```python
from build123d import *

# Parameters (mm, degrees)
SKETCH3_W           = 156.772980402
SKETCH3_H           = 60
BOSS_EXTRUDE6_DEPTH = 12
CUT_EXTRUDE1_REACH  = 14
SKETCH4_R           = 2.25
CUT_EXTRUDE2_REACH  = 14
SKETCH6_R           = 3.25
SKETCH7_R           = 3.5
CUT_EXTRUDE3_DEPTH  = 5
SKETCH8_R           = 5
CUT_EXTRUDE4_DEPTH  = 7
CUT_EXTRUDE5_REACH  = 14
SKETCH9_R           = 2.75


with BuildPart() as part:
    # Sketch3 → Boss-Extrude6 (new body)
    with BuildSketch(Plane(origin=(-27.52701042, 0, 0), x_dir=(0, 0, 1), z_dir=(0, 1, 0))):
        with Locations((-23.695908121, 17.809773729)):
            Rectangle(SKETCH3_W, SKETCH3_H)
    extrude(amount=BOSS_EXTRUDE6_DEPTH)

    # Sketch4 → Cut-Extrude1 (cut, up to next)
    with BuildSketch(Plane(origin=(0, 12, 0), x_dir=(1, 0, 0), z_dir=(0, 1, 0)), mode=Mode.PRIVATE) as cut_extrude1_sk1:
        with Locations((-1.126993796, -19.304091879)):
            Circle(SKETCH4_R)
    cut_extrude1_tool1 = extrude(cut_extrude1_sk1.sketch, amount=-CUT_EXTRUDE1_REACH, mode=Mode.PRIVATE) & part.part
    add(cut_extrude1_tool1.solids().sort_by_distance((-1.126994, 12, 19.304092))[0], mode=Mode.SUBTRACT)
    # Sketch4 → Cut-Extrude1 (cut, up to next)
    with BuildSketch(Plane(origin=(0, 12, 0), x_dir=(1, 0, 0), z_dir=(0, 1, 0)), mode=Mode.PRIVATE) as cut_extrude1_sk2:
        with Locations((-19.127096376, -19.304091879)):
            Circle(SKETCH4_R)
    cut_extrude1_tool2 = extrude(cut_extrude1_sk2.sketch, amount=-CUT_EXTRUDE1_REACH, mode=Mode.PRIVATE) & part.part
    add(cut_extrude1_tool2.solids().sort_by_distance((-19.127096, 12, 19.304092))[0], mode=Mode.SUBTRACT)
    # Sketch4 → Cut-Extrude1 (cut, up to next)
    with BuildSketch(Plane(origin=(0, 12, 0), x_dir=(1, 0, 0), z_dir=(0, 1, 0)), mode=Mode.PRIVATE) as cut_extrude1_sk3:
        with Locations((-1.2080193, -43.304091879)):
            Circle(SKETCH4_R)
    cut_extrude1_tool3 = extrude(cut_extrude1_sk3.sketch, amount=-CUT_EXTRUDE1_REACH, mode=Mode.PRIVATE) & part.part
    add(cut_extrude1_tool3.solids().sort_by_distance((-1.208019, 12, 43.304092))[0], mode=Mode.SUBTRACT)
    # Sketch4 → Cut-Extrude1 (cut, up to next)
    with BuildSketch(Plane(origin=(0, 12, 0), x_dir=(1, 0, 0), z_dir=(0, 1, 0)), mode=Mode.PRIVATE) as cut_extrude1_sk4:
        with Locations((-19.208121879, -43.304091879)):
            Circle(SKETCH4_R)
    cut_extrude1_tool4 = extrude(cut_extrude1_sk4.sketch, amount=-CUT_EXTRUDE1_REACH, mode=Mode.PRIVATE) & part.part
    add(cut_extrude1_tool4.solids().sort_by_distance((-19.208122, 12, 43.304092))[0], mode=Mode.SUBTRACT)
    # Sketch4 → Cut-Extrude1 (cut, up to next)
    with BuildSketch(Plane(origin=(0, 12, 0), x_dir=(1, 0, 0), z_dir=(0, 1, 0)), mode=Mode.PRIVATE) as cut_extrude1_sk5:
        with Locations((-19.208121879, 66.695908121)):
            Circle(SKETCH4_R)
    cut_extrude1_tool5 = extrude(cut_extrude1_sk5.sketch, amount=-CUT_EXTRUDE1_REACH, mode=Mode.PRIVATE) & part.part
    add(cut_extrude1_tool5.solids().sort_by_distance((-19.208122, 12, -66.695908))[0], mode=Mode.SUBTRACT)
    # Sketch4 → Cut-Extrude1 (cut, up to next)
    with BuildSketch(Plane(origin=(0, 12, 0), x_dir=(1, 0, 0), z_dir=(0, 1, 0)), mode=Mode.PRIVATE) as cut_extrude1_sk6:
        with Locations((-19.208121879, 90.695908121)):
            Circle(SKETCH4_R)
    cut_extrude1_tool6 = extrude(cut_extrude1_sk6.sketch, amount=-CUT_EXTRUDE1_REACH, mode=Mode.PRIVATE) & part.part
    add(cut_extrude1_tool6.solids().sort_by_distance((-19.208122, 12, -90.695908))[0], mode=Mode.SUBTRACT)
    # Sketch4 → Cut-Extrude1 (cut, up to next)
    with BuildSketch(Plane(origin=(0, 12, 0), x_dir=(1, 0, 0), z_dir=(0, 1, 0)), mode=Mode.PRIVATE) as cut_extrude1_sk7:
        with Locations((-1.2080193, 90.695908121)):
            Circle(SKETCH4_R)
    cut_extrude1_tool7 = extrude(cut_extrude1_sk7.sketch, amount=-CUT_EXTRUDE1_REACH, mode=Mode.PRIVATE) & part.part
    add(cut_extrude1_tool7.solids().sort_by_distance((-1.208019, 12, -90.695908))[0], mode=Mode.SUBTRACT)
    # Sketch4 → Cut-Extrude1 (cut, up to next)
    with BuildSketch(Plane(origin=(0, 12, 0), x_dir=(1, 0, 0), z_dir=(0, 1, 0)), mode=Mode.PRIVATE) as cut_extrude1_sk8:
        with Locations((-1.2080193, 66.695908121)):
            Circle(SKETCH4_R)
    cut_extrude1_tool8 = extrude(cut_extrude1_sk8.sketch, amount=-CUT_EXTRUDE1_REACH, mode=Mode.PRIVATE) & part.part
    add(cut_extrude1_tool8.solids().sort_by_distance((-1.208019, 12, -66.695908))[0], mode=Mode.SUBTRACT)

    # Sketch6 → Cut-Extrude2 (cut, up to next)
    with BuildSketch(Plane(origin=(0, 12, 0), x_dir=(1, 0, 0), z_dir=(0, 1, 0)), mode=Mode.PRIVATE) as cut_extrude2_sk1:
        with Locations((-17.217236691, 18.631632081)):
            Circle(SKETCH6_R)
    cut_extrude2_tool1 = extrude(cut_extrude2_sk1.sketch, amount=-CUT_EXTRUDE2_REACH, mode=Mode.PRIVATE) & part.part
    add(cut_extrude2_tool1.solids().sort_by_distance((-17.217237, 12, -18.631632))[0], mode=Mode.SUBTRACT)
    # Sketch6 → Cut-Extrude2 (cut, up to next)
    with BuildSketch(Plane(origin=(0, 12, 0), x_dir=(1, 0, 0), z_dir=(0, 1, 0)), mode=Mode.PRIVATE) as cut_extrude2_sk2:
        with Locations((-2.217236691, 18.631632081)):
            Circle(SKETCH6_R)
    cut_extrude2_tool2 = extrude(cut_extrude2_sk2.sketch, amount=-CUT_EXTRUDE2_REACH, mode=Mode.PRIVATE) & part.part
    add(cut_extrude2_tool2.solids().sort_by_distance((-2.217237, 12, -18.631632))[0], mode=Mode.SUBTRACT)

    # Sketch7 → Cut-Extrude3 (cut)
    with BuildSketch(Plane(origin=(0, 12, 0), x_dir=(1, 0, 0), z_dir=(0, 1, 0))):
        with Locations((-19.127096376, -19.304091879)):
            Circle(SKETCH7_R)
        with Locations((-19.208121879, -43.304091879)):
            Circle(SKETCH7_R)
        with Locations((-1.2080193, -43.304091879)):
            Circle(SKETCH7_R)
        with Locations((-1.126993796, -19.304091879)):
            Circle(SKETCH7_R)
        with Locations((-1.2080193, 66.695908121)):
            Circle(SKETCH7_R)
        with Locations((-19.208121879, 66.695908121)):
            Circle(SKETCH7_R)
        with Locations((-19.208121879, 90.695908121)):
            Circle(SKETCH7_R)
        with Locations((-1.2080193, 90.695908121)):
            Circle(SKETCH7_R)
    extrude(amount=-CUT_EXTRUDE3_DEPTH, mode=Mode.SUBTRACT)

    # Sketch8 → Cut-Extrude4 (cut)
    with BuildSketch(Plane(origin=(0, 12, 0), x_dir=(1, 0, 0), z_dir=(0, 1, 0))):
        with Locations((-17.217236691, 18.631632081)):
            Circle(SKETCH8_R)
        with Locations((-2.217236691, 18.631632081)):
            Circle(SKETCH8_R)
    extrude(amount=-CUT_EXTRUDE4_DEPTH, mode=Mode.SUBTRACT)

    # Sketch9 → Cut-Extrude5 (cut, up to next)
    with BuildSketch(Plane(origin=(0, 12, 0), x_dir=(1, 0, 0), z_dir=(0, 1, 0)), mode=Mode.PRIVATE) as cut_extrude5_sk1:
        with Locations((-31.657880115, 23.701844607)):
            Circle(SKETCH9_R)
    cut_extrude5_tool1 = extrude(cut_extrude5_sk1.sketch, amount=-CUT_EXTRUDE5_REACH, mode=Mode.PRIVATE) & part.part
    add(cut_extrude5_tool1.solids().sort_by_distance((-31.65788, 12, -23.701845))[0], mode=Mode.SUBTRACT)
    # Sketch9 → Cut-Extrude5 (cut, up to next)
    with BuildSketch(Plane(origin=(0, 12, 0), x_dir=(1, 0, 0), z_dir=(0, 1, 0)), mode=Mode.PRIVATE) as cut_extrude5_sk2:
        with Locations((14.282732382, 23.735684254)):
            Circle(SKETCH9_R)
    cut_extrude5_tool2 = extrude(cut_extrude5_sk2.sketch, amount=-CUT_EXTRUDE5_REACH, mode=Mode.PRIVATE) & part.part
    add(cut_extrude5_tool2.solids().sort_by_distance((14.282732, 12, -23.735684))[0], mode=Mode.SUBTRACT)


solid = part.part
```
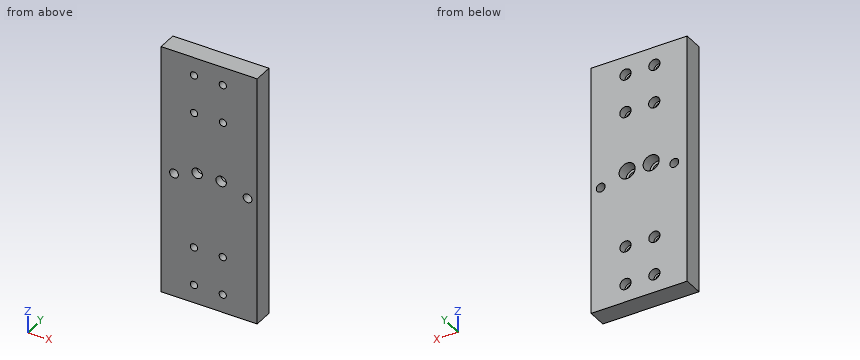
Work out the finished part from the listing and answer in its coordinate system (mm). Round coordinates to 2 decimals unless told otherwise and drop trailing zeros.
1) Consider probe 1 along Z at (x, y) = (-6, 10.5); probe 2 along X at (y, z) = (10.75, -25); probe 3 along Z at (x, y) = (-17, 7.5). Determine where each line is inside the solid, lowest interval first.
2) Flat-ended cylindrical pins translate along their axes: P1, Ø3, axis at x = 0, z = -19, coming from the +Y side; P2, Ø4, axis at x = -23, z = -25.5, coming from the -Y side; P3, Ø6, axis at x = -19.13, z = 19.3, coming from the +Y side. Find the tip coordinate at first contact, or state that the pin passes through.
3) A cutting plane is placed at A-A on y = 10. Give the number of separate pieces and of enclosed holes in the cut face, and give its area (3 significant figures).
Entries:
1. probe 1: z = -102.08 to -21.9, -15.36 to 54.69
1. probe 2: x = -39.72 to -34.08, -29.23 to 11.84, 16.72 to 20.28
1. probe 3: z = -102.08 to -93.41, -87.98 to -69.41, -63.98 to -23.63, -13.64 to 16.52, 22.08 to 40.59, 46.02 to 54.69
2. P1: stops at y = 5
2. P2: stops at y = 0
2. P3: stops at y = 7
3. separate pieces: 1
3. enclosed holes: 12
3. area: 8,890 mm2
